```python
from build123d import *


with BuildPart() as part:
    # Sketch1 → Revolve1 (revolve)
    with BuildSketch(Plane(origin=(0, 0, 0), x_dir=(1, 0, 0), z_dir=(0, 1, 0)), mode=Mode.PRIVATE) as revolve1_sk:
        with BuildLine():
            Line((0, 0), (0, 2))
            ThreePointArc((0, 2), (0.03579799, 2.086424), (0.122221986, 2.122222))
            Line((0.122221986, 2.122222), (1.377777546, 2.122222))
            ThreePointArc((1.377777546, 2.122222), (1.464201541, 2.086424015), (1.499999546, 2.000000028))
            Line((1.499999546, 2.000000028), (1.5, 2.8e-08))
            ThreePointArc((1.5, 2.8e-08), (1.46420195, -0.086424151), (1.37777778, -0.12222222))
            Line((1.37777778, -0.12222222), (0.12222222, -0.12222222))
            ThreePointArc((0.12222222, -0.12222222), (0.035798059, -0.086424161), (0, 0))
        make_face()
    revolve(revolve1_sk.sketch.rotate(Axis((-1.5, 0, -2), (0, 0, 1)), 180), axis=Axis((-1.5, 0, -2), (0, 0, 1)))


solid = part.part
```
Can you work these out from the model? Positions are in its coordinate system, mm. Give positions to 0.01 mm unless a question says otherwise; leave off trailing zeros. Write each loop counter-clockwise with the first axis right and the second up, starting at its lowest first coordinate (ties: lowest second). Pieces come first, ordered by that corner, then holes. Notation, with made-up numbers: (-38, -23) -> (-22, -23) arc R35 cw to (-22, 16) -> close; hole circle Ø1 at (-28.5, 24). An arc over 180 degrees is marked (long way). Write item = value, one per line.
(1) I need wall thicknesses on probe 1 along Y at (x, z) = (-1.5, -0.55); probe 2 along Y at (x, z) = (-2.25, -1.5); probe 3 along Z at (x, y) = (-0.25, 1). Which ranges of each line are inside material? Lowest first, please. Write a range as from..to.
Worked out:
probe_1 = -3..-1.5, 1.5..3
probe_2 = -2.9..-1.3, 1.3..2.9
probe_3 = -2.12..0.12
(2) Suppose I cut it at B-B on z = -0.7. Write out the boundary of the cut face in (x, y), then the cut area to 3 significant figures.
Worked out:
outline = circle Ø6 at (-1.5, 0); hole circle Ø3 at (-1.5, 0)
area = 21.2 mm^2
(3) Thinking about a two-plate mould opening in X: for faces 1 (the face through (0.9, 1.8, -1)), 2 (the face through (0, 1, -2.122)), 3 (the face through (0, 0, -1)), which applies, released by +X, released by -X, zero draft, split by the parting line, or undercut?
Worked out:
face_1 = split by the parting line
face_2 = zero draft
face_3 = undercut
(4) Suppose I cut it at A-A on x = -1.5. Write out the boundary of the cut face in (y, z), then the cut area to 3 significant figures.
Worked out:
outline = (-3, -2) arc R0.12 ccw to (-2.88, -2.12) -> (-1.62, -2.12) arc R0.12 ccw to (-1.5, -2) -> (-1.5, 0) arc R0.12 ccw to (-1.62, 0.12) -> (-2.88, 0.12) arc R0.12 ccw to (-3, 0) -> close; (1.5, -2) arc R0.12 ccw to (1.62, -2.12) -> (2.88, -2.12) arc R0.12 ccw to (3, -2) -> (3, 0) arc R0.12 ccw to (2.88, 0.12) -> (1.62, 0.12) arc R0.12 ccw to (1.5, 0) -> close
area = 6.71 mm^2
(5) I'm going to push flat-ended pins straight in: P1, Ø3.5, axis at x = -1.5, y = 0, coming from the +Z side; P2, Ø1, axis at x = 0, z = -2, coming from the +Y side. Where does each tip first touch, or does it pass through?
Worked out:
P1 = 0.12
P2 = 2.83
